For this review, take the finished solid that the model builds, in its own axes (mm). Round coordinates to 2 decimals unless told otherwise and drop trailing zeros. One line per question, with ' | ' between items.
```python
from build123d import *

# Parameters (mm, degrees)
STRUCTURAL_MEMBER2_DEPTH = 525


with BuildPart() as part:
    # Profile → Structural Member2 (new body)
    with BuildSketch(Plane(origin=(0, 0, 0), x_dir=(0, 0, -1), z_dir=(1, 0, 0))):
        with BuildLine():
            Line((69.699997, 55), (64.5, 55))
            Line((64.5, 55), (64.5, 60))
            Line((64.5, 60), (61.767777, 60))
            Line((61.767777, 60), (57.5, 55.732231))
            Line((57.5, 55.732231), (57.5, 50.519615242))
            Line((57.5, 50.519615242), (57.2, 50))
            Line((57.2, 50), (57.5, 49.480384758))
            Line((57.5, 49.480384758), (57.5, 44.26777))
            Line((57.5, 44.26777), (61.767777, 39.999999))
            Line((61.767777, 39.999999), (64.5, 40))
            Line((64.5, 40), (64.5, 45))
            Line((64.5, 45), (69.699997, 45))
            ThreePointArc((69.699997, 45), (69.912132034, 44.912132034), (70, 44.699997))
            Line((70, 44.699997), (70, 33))
            ThreePointArc((70, 33), (69.121320344, 30.878679656), (67, 30))
            Line((67, 30), (55.3, 30))
            ThreePointArc((55.3, 30), (55.087867966, 30.087867966), (55, 30.3))
            Line((55, 30.3), (55, 35.5))
            Line((55, 35.5), (60, 35.5))
            Line((60, 35.5), (60.000008, 38.232225))
            Line((60.000008, 38.232225), (55.732238, 42.5))
            Line((55.732238, 42.5), (50.519615242, 42.5))
            Line((50.519615242, 42.5), (50, 42.8))
            Line((50, 42.8), (49.480384758, 42.5))
            Line((49.480384758, 42.5), (44.26777, 42.5))
            Line((44.26777, 42.5), (40, 38.23223))
            Line((40, 38.23223), (40, 35.5))
            Line((40, 35.5), (45, 35.5))
            Line((45, 35.5), (45, 30.3))
            ThreePointArc((45, 30.3), (44.912130974, 30.087866905), (44.699997, 30))
            Line((44.699997, 30), (33, 30))
            ThreePointArc((33, 30), (30.878679656, 30.878679656), (30, 33))
            Line((30, 33), (30, 44.699997))
            ThreePointArc((30, 44.699997), (30.087867966, 44.912132034), (30.300003, 45))
            Line((30.300003, 45), (35.5, 45))
            Line((35.5, 45), (35.5, 40.000006))
            Line((35.5, 40.000006), (38.232224, 40.000006))
            Line((38.232224, 40.000006), (42.5, 44.267753))
            Line((42.5, 44.267753), (42.5, 49.480384758))
            Line((42.5, 49.480384758), (42.8, 50))
            Line((42.8, 50), (42.5, 50.519615242))
            Line((42.5, 50.519615242), (42.5, 55.732248))
            Line((42.5, 55.732248), (38.232231, 60.000001))
            Line((38.232231, 60.000001), (35.5, 60))
            Line((35.5, 60), (35.5, 55))
            Line((35.5, 55), (30.300003, 55))
            ThreePointArc((30.300003, 55), (30.087867966, 55.087867966), (30, 55.300003))
            Line((30, 55.300003), (30, 67.000001))
            ThreePointArc((30, 67.000001), (30.87868001, 69.121320697), (33, 70))
            Line((33, 70), (44.699997, 70))
            ThreePointArc((44.699997, 70), (44.912130974, 69.912133095), (45, 69.7))
            Line((45, 69.7), (45, 64.5))
            Line((45, 64.5), (40, 64.5))
            Line((40, 64.5), (40, 61.767771))
            Line((40, 61.767771), (44.267771, 57.5))
            Line((44.267771, 57.5), (49.480384758, 57.5))
            Line((49.480384758, 57.5), (50, 57.2))
            Line((50, 57.2), (50.519615242, 57.5))
            Line((50.519615242, 57.5), (55.732237, 57.5))
            Line((55.732237, 57.5), (60.000008, 61.767771))
            Line((60.000008, 61.767771), (60, 64.5))
            Line((60, 64.5), (55, 64.5))
            Line((55, 64.5), (55, 69.7))
            ThreePointArc((55, 69.7), (55.087867966, 69.912132034), (55.3, 70))
            Line((55.3, 70), (67, 70))
            ThreePointArc((67, 70), (69.12131999, 69.121320697), (70, 67.000001))
            Line((70, 67.000001), (70, 55.300003))
            ThreePointArc((70, 55.300003), (69.912132034, 55.087867966), (69.699997, 55))
        make_face()
        with BuildLine():
            Line((37, 68), (33, 68))
            ThreePointArc((33, 68), (32.292893219, 67.707106781), (32, 67))
            Line((32, 67), (32, 63))
            ThreePointArc((32, 63), (32.292893219, 62.292893219), (33, 62))
            Line((33, 62), (37, 62))
            ThreePointArc((37, 62), (37.707106781, 62.292893219), (38, 63))
            Line((38, 63), (38, 67))
            ThreePointArc((38, 67), (37.707106781, 67.707106781), (37, 68))
        make_face(mode=Mode.SUBTRACT)
        with BuildLine():
            Line((68, 67), (68, 63))
            ThreePointArc((68, 63), (67.707106781, 62.292893219), (67, 62))
            Line((67, 62), (62.999985, 62))
            ThreePointArc((62.999985, 62), (62.29288933, 62.292897108), (62, 62.999996))
            Line((62, 62.999996), (62, 67))
            ThreePointArc((62, 67), (62.292893219, 67.707106781), (63, 68))
            Line((63, 68), (67, 68))
            ThreePointArc((67, 68), (67.707106781, 67.707106781), (68, 67))
        make_face(mode=Mode.SUBTRACT)
        with BuildLine():
            Line((68, 33), (68, 37.000001))
            ThreePointArc((68, 37.000001), (67.707106781, 37.707107781), (67, 38.000001))
            Line((67, 38.000001), (63, 38.000001))
            ThreePointArc((63, 38.000001), (62.292893219, 37.707107781), (62, 37.000001))
            Line((62, 37.000001), (62, 33))
            ThreePointArc((62, 33), (62.292893219, 32.292893219), (63, 32))
            Line((63, 32), (67, 32))
            ThreePointArc((67, 32), (67.707106781, 32.292893219), (68, 33))
        make_face(mode=Mode.SUBTRACT)
        with BuildLine():
            Line((33, 38), (37.000015, 38))
            ThreePointArc((37.000015, 38), (37.707114206, 37.707099357), (38, 36.999994))
            Line((38, 36.999994), (38, 33))
            ThreePointArc((38, 33), (37.707106781, 32.292893219), (37, 32))
            Line((37, 32), (33, 32))
            ThreePointArc((33, 32), (32.292893219, 32.292893219), (32, 33))
            Line((32, 33), (32, 37))
            ThreePointArc((32, 37), (32.292893219, 37.707106781), (33, 38))
        make_face(mode=Mode.SUBTRACT)
        with BuildLine():
            ThreePointArc((45.693983688, 53.003451934), (44.75, 50.000006422), (45.69397634, 46.996558601))
            ThreePointArc((45.69397634, 46.996558601), (45.717617411, 46.612262817), (45.393937878, 46.403759319))
            ThreePointArc((45.393937878, 46.403759319), (44.696798004, 44.696601447), (46.403759064, 45.394223081))
            ThreePointArc((46.403759064, 45.394223081), (46.613183993, 45.71810041), (46.998050321, 45.692936253))
            ThreePointArc((46.998050321, 45.692936253), (50.001173377, 44.750000131), (53.00387464, 45.694278557))
            ThreePointArc((53.00387464, 45.694278557), (53.38786573, 45.717565842), (53.596237266, 45.39418873))
            ThreePointArc((53.596237266, 45.39418873), (55.303208824, 44.696612273), (54.60606185, 46.403759282))
            ThreePointArc((54.60606185, 46.403759282), (54.2823423, 46.612342937), (54.306127195, 46.996707043))
            ThreePointArc((54.306127195, 46.996707043), (55.25, 50.000037648), (54.306084121, 53.003354715))
            ThreePointArc((54.306084121, 53.003354715), (54.28277906, 53.388519532), (54.607953771, 53.596260884))
            ThreePointArc((54.607953771, 53.596260884), (55.30278657, 55.303809323), (53.596244226, 54.606509157))
            ThreePointArc((53.596244226, 54.606509157), (53.387865247, 54.28245073), (53.003318835, 54.306109146))
            ThreePointArc((53.003318835, 54.306109146), (50.000075464, 55.249999999), (46.996804959, 54.306195484))
            ThreePointArc((46.996804959, 54.306195484), (46.612495539, 54.2822647), (46.403758539, 54.605831196))
            ThreePointArc((46.403758539, 54.605831196), (44.696618996, 55.30321925), (45.394389581, 53.596236026))
            ThreePointArc((45.394389581, 53.596236026), (45.717718991, 53.387547534), (45.693983688, 53.003451934))
        make_face(mode=Mode.SUBTRACT)
    extrude(amount=STRUCTURAL_MEMBER2_DEPTH)


solid = part.part
```
Item 1: Take a section at A-A (x = 84). State how many separate pieces and enclosed holes the cut face has, then the cut area to 3 significant figures.
Results:
separate pieces: 1 | enclosed holes: 5 | area: 643 mm2
Item 2: Insertion check: pin 1 Ø8 at (y, z) = (36.5, -40) entering from -X; pin 2 Ø6 at (x, z) = (113, -48.5) entering from -Y. Each pin has a flat end and moves straight along its axis. Give the tip position at first contact, or say it passes through.
Results:
pin 1: x = 0 | pin 2: y = 42.5
Item 3: To check wall thickness, follow line 1 along Z through (x, y) = (432, 34.5); line 2 along Y through (x, z) = (269.5, -34); line 3 along Y through (x, z) = (412, -37). State the ranges of each line that lie inside material, in increasing order. Write a range as from..to.
Results:
line 1: -70..-68, -62..-55, -45..-38, -32..-30 | line 2: 30..32, 38..45, 55..62, 68..70 | line 3: 30..32, 38..40, 60..62, 68..70
